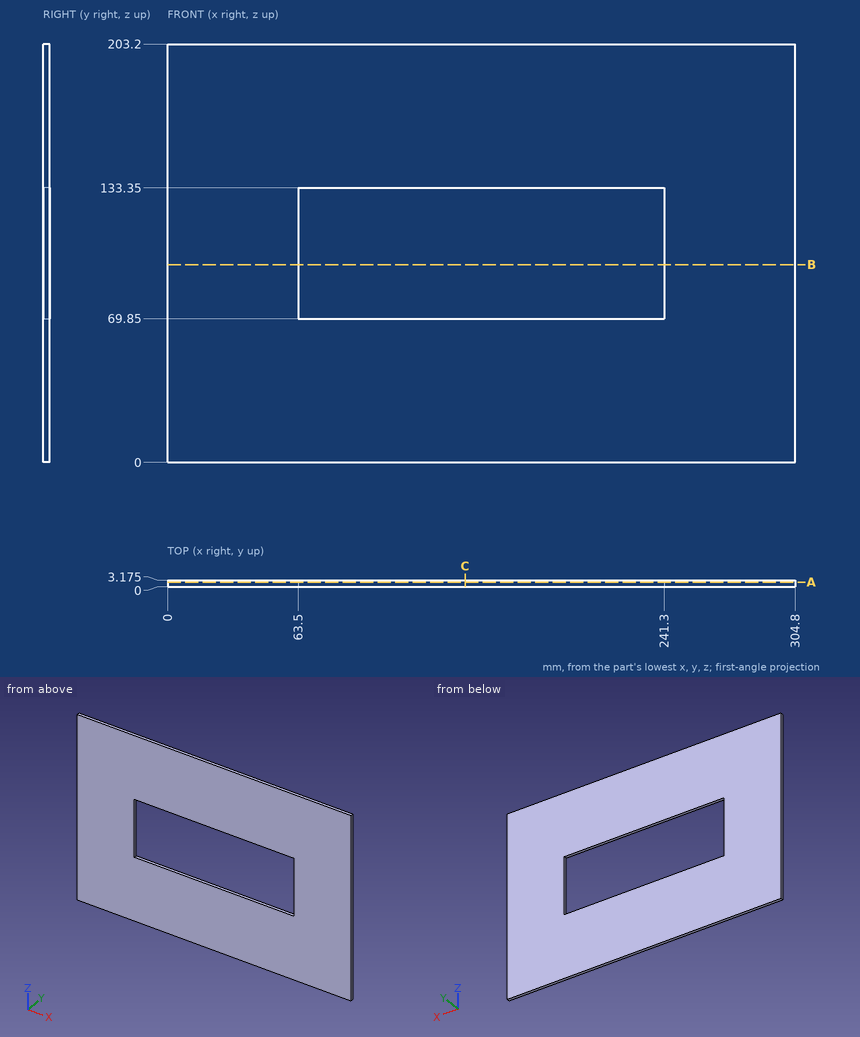
Can you work these out from the drawing? Everything is in mm from the part's minimum corner. Round coordinates to 2 decimals unless told otherwise and drop trailing zeros. Write each loop counter-clockwise with the first axis right and the second up, starting at its lowest first coordinate (ties: lowest second). Pieces come first, ordered by that corner, then holes.
1. Suppose I cut it at A-A (y = 2.35). List the corners of the cut face in (x, z) for me, and give its area (3 significant figures).
2. Suppose I cut it at C-C (x = 144.5). List the corners of the cut face in (y, z) for me (3 decimals).
3. I need wall thicknesses on L1, parallel to Z at x = 64, y = 1.25; L2, parallel to X at y = 1.8, z = 94.5. Which ranges of each line are inside material? Lowest first, please.
4. Will this pin go through, and if not, where does the flat tip stop? pin 1 Ø1 at (y, z) = (1, 117) entering from -X.
5. Suppose I cut it at B-B (z = 96). List the corners of the cut face in (x, y) for me (3 decimals), and give its area (3 significant figures).
Answer sheet:
1. outline: (0, 0) - (304.8, 0) - (304.8, 203.2) - (0, 203.2) - close; hole (63.5, 69.85) - (241.3, 69.85) - (241.3, 133.35) - (63.5, 133.35) - close
1. area: 50,600 mm2
2. outline: (0, 0) - (3.175, 0) - (3.175, 69.85) - (0, 69.85) - close; (0, 133.35) - (3.175, 133.35) - (3.175, 203.2) - (0, 203.2) - close
3. L1: z = 0 to 69.85, 133.35 to 203.2
3. L2: x = 0 to 63.5, 241.3 to 304.8
4. pin 1: stops at x = 0
5. outline: (0, 0) - (63.5, 0) - (63.5, 3.175) - (0, 3.175) - close; (241.3, 0) - (304.8, 0) - (304.8, 3.175) - (241.3, 3.175) - close
5. area: 403 mm2
